For this review, take the finished solid that the model builds, in its own axes (mm). Face numbers are marked on the shaded views. A direction names the side the tool comes from. Coordinates: 2 decimals unless noted, no trailing zeros. Loops run counter-clockwise (first coordinate to the right, second up) from the corner with the lowest first, then second, coordinate; pieces in that order, holes last. Notation, with made-up numbers: M 65,-17 L 82,-17 A19 ccw 82,-13 Z; hole C 15,68.25 d4. An arc over 180 degrees is marked long. Answer as a JSON object with one key per item and string values. Group by question number.
Item 1: Add section A-A (x = 35). State the section outline as (y, z) points.
Item 2: Tool access review of the marked faces 1 and 2: name each direction out of +Z, -Z, +X, -X, +Y, -Y from which nothing blocks a thin tool from reaching the whole face with its end or side.
Item 3: Insertion check: pin 1 (1.5 mm diameter, centred on x = 58.5, y = 2.5, fed in from +Z); pin 2 (1.5 mm diameter, centred on x = 53.5, y = -3, fed in from +Z); pin 3 (1.5 mm diameter, centred on x = 49, z = 3.5, fed in from -Y). Each pin has a flat end and moves straight along its axis. Give the tip position at first contact, or say it passes through.
Item 4: Wall thickness on L1, parallel to X at y = -3, z = -5.75; L2, parallel to Y at x = 36.5, z = 0; L3, parallel to Z at x = 1.5, y = -0.25: over which ranges is each line inside the solid? List them lowest first. Write a range as from..to.
Autodesk Inventor part; units mm, degrees
ref_plane "Work Plane1" through (1.525, 0, 0) normal (0, 0, 1) x (1, 0, 0)
ref_plane "YZ Plane" through (0, 0, 0) normal (1, 0, 0) x (0, 1, 0)
ref_plane "XZ Plane" through (0, 0, 0) normal (0, 1, 0) x (-1, 0, 0)
sketch "Sketch1" plane through (0, 0, 0) normal (0, 0, 1) x (1, 0, 0)
  line L0 (0, 4) -> (70, 4)
  line L1 (70, 4) -> (70, 0)
  line L2 (70, 0) -> (0, 0)
  line L3 (-17, 0) -> (102, 0)
  line L4 (0, -0.8) -> (0, 4.8)
  line L5 (0, 4) -> (0, 0)
  dimension "d2" = 8
  dimension "d59" = 70
revolve "Body" add sketch "Sketch1" angle 360 about axis through (70, 0, 0) along (-1, 0, 0)
sketch "Sketch2" plane through (0, 0, 0) normal (-1, 0, 0) x (0, 0, 1)
  line L0 (0, 7.5056) -> (6.5, 3.7528)
  line L1 (6.5, 3.7528) -> (6.5, -3.7528)
  line L2 (6.5, -3.7528) -> (0, -7.5056)
  line L3 (0, -7.5056) -> (-6.5, -3.7528)
  line L4 (-6.5, -3.7528) -> (-6.5, 3.7528)
  line L5 (-6.5, 3.7528) -> (0, 7.5056)
  line L6 (-9.1, 0) -> (9.1, 0)
  line L7 (0, 10.5078) -> (0, -10.5078)
  point P0 (0, 0)
  point P1 (0, 0)
  dimension "d11" = 13
extrude "Head" add sketch "Sketch2" along normal blind 5.68
sketch "Sketch4" plane through (0, 0, 0) normal (0, 0, 1) x (1, 0, 0)
  line L0 (-4.9294, 7.8) -> (-5.68, 6.5)
  line L1 (-1.1, 0) -> (-0.234, 0)
  line L2 (-6.7692, 0) -> (0.8552, 0)
  line L3 (-5.68, 7.8) -> (-4.9294, 7.8)
  line L4 (-5.68, 6.5) -> (-5.68, 7.8)
  line L5 (0, 9.36) -> (0, -1.56)
  dimension "d65" = 13
  dimension "d67" = 30
  dimension "d68" = 15.6
  dimension "d69" = 5.68
revolve "Chamfer1" cut sketch "Sketch4" angle 360 about axis through (-1.1, 0, 0) along (1, 0, 0)
thread "Thread"
chamfer "Chamfer2" distance 0.7668 distance2 0.7669 1 edges at (70, -4, 0) measured on face at (70, 1.3909, 1.1742)
fillet "Fillet" radius 0.1 1 edges at (0, -4, 0)
ref_plane "Work Plane1" through (1.525, 0, 0) normal (0, 0, 1) x (1, 0, 0)
equation "\"d2\" = GD"
equation "\"d59\" = NLG"
equation "\"d11\" = SW"
equation "\"d3\" = KOH"
equation "\"d15\" = GEL"
equation "\"d6\" = -0.5 * SPD + 0.5 * GD"
equation "\"d71\" = RR"
equation "\"d65\" = SW"
equation "\"d67\" = ANG1"
equation "\"d68\" = 1.2 * SW"
equation "\"d69\" = KOH"
equation "\"NLG\" = 70"
equation "\"GD\" = NND"
equation "\"BDM\" = NND"
equation "\"KOH\" = 5.68"
equation "\"GEL\" = 22"
equation "\"SW\" = 13"
equation "\"SW0\" = SW"
equation "\"SPD\" = NND - 1.2269 * PTC"
equation "\"SD2\" = NND"
equation "\"SD\" = 0"
equation "\"ANG1\" = 30deg"
equation "\"GAL\" = 0.61345 * PTC"
equation "\"GUL\" = 0.61345 * PTC"
equation "\"RR\" = 0.1"
equation "\"RR1\" = 0.4"
equation "\"GD1\" = THREADDIA - 1.2269 * PTC"
equation "\"THREADDIA\" = 8"
equation "\"TOA\" = 30deg"
equation "\"PTC\" = 1.25"
equation "\"KOH1\" = 3.7"
equation "\"NND\" = 8"
equation "\"E0\" = 1.155 * SW"
properties part number "ANSI B18.2.3.5M - M8 x 1.25 x 70" material "Steel, Mild"
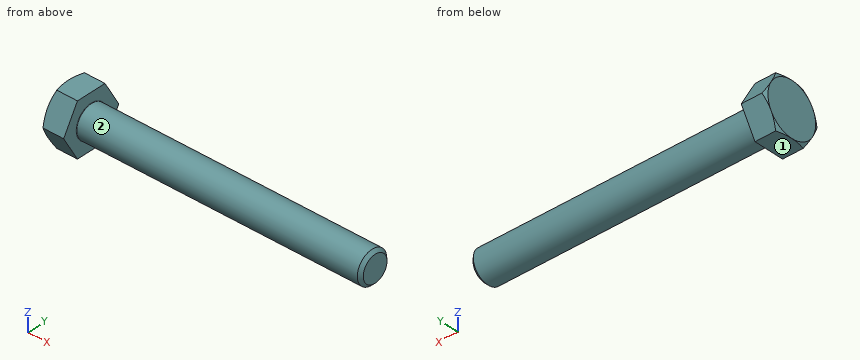
From the geometry:
{
 "1": {"outline": "C 0,0 d8"},
 "2": {"face 1": "-Z, +X, -X, +Y, -Y", "face 2": "+X"},
 "3": {"pin 1": "stops at z = 3.6", "pin 2": "stops at z = 3.31", "pin 3": "stops at y = -2.9"},
 "4": {"L1": "x = -5.68..0", "L2": "y = -4..4", "L3": "z = -3.99..3.99"}
}
